The listing builds one solid part. Answer for the finished solid, in the listing's coordinates (mm). A direction names the side the tool comes from. Give positions to 0.01 mm unless a question says otherwise; leave off trailing zeros. Order: outer loops, then holes, each group sorted by start corner. A loop starts at its lowest first (then second) coordinate and runs counter-clockwise, first axis right, second up.
```python
from build123d import *

# Parameters (mm, degrees)
F1_DEPTH       = 35
F3_D           = 5
F3_START       = 1.8205079
F3_CBORE_D     = 10
F3_CBORE_DEPTH = 8
F4_W           = 22.5
F4_H           = 2
F5_DEPTH       = 25
F6_R           = 6
F7_DEPTH       = 8


with BuildPart() as f1:
    # F0 (on Top) → F1 (new body, symmetric)
    with BuildSketch(Plane.XY):
        with BuildLine():
            ThreePointArc((-17.3192642082, 2.5086026559), (17.5, 0), (-17.3192642082, -2.5086026559))
            Line((-17.3192642082, -2.5086026559), (-28.1192642082, -2.5086026559))
            Line((-28.1192642082, -2.5086026559), (-28.1192642082, -10.9086026559))
            ThreePointArc((-28.1192642082, -10.9086026559), (-25.7761184577, -16.5654569054), (-20.1192642082, -18.9086026559))
            Line((-20.1192642082, -18.9086026559), (-7.9192642082, -18.9086026559))
            ThreePointArc((-7.9192642082, -18.9086026559), (20.5, 0), (-7.9192642082, 18.9086026559))
            Line((-7.9192642082, 18.9086026559), (-20.1192642082, 18.9086026559))
            ThreePointArc((-20.1192642082, 18.9086026559), (-25.7761184577, 16.5654569054), (-28.1192642082, 10.9086026559))
            Line((-28.1192642082, 10.9086026559), (-28.1192642082, 2.5086026559))
            Line((-28.1192642082, 2.5086026559), (-17.3192642082, 2.5086026559))
        make_face()
    extrude(amount=F1_DEPTH, both=True)

    # F3 (through all)
    # its depths count from where the whole tool has entered the part; down to there all is cleared
    with Locations(Plane.XZ.offset(18.9086026559).offset(-F3_START)):
        with Locations((-20.2, 24.25), (-20.2, 9.25), (-20.2, -9.25), (-20.2, -24.25)):
            CounterBoreHole(F3_D / 2, F3_CBORE_D / 2, F3_CBORE_DEPTH)

    # F4 (on Front) → F5 (cut, symmetric)
    with BuildSketch(Plane.XZ):
        with Locations((-11.25, 0)):
            Rectangle(F4_W, F4_H)
    extrude(amount=F5_DEPTH, both=True, mode=Mode.SUBTRACT)

    # F6 (on Top) → F7 (cut)
    with BuildSketch(Plane.XY):
        with Locations((0, -25)):
            Circle(F6_R)
        with Locations((17.6776695297, -17.6776695297)):
            Circle(F6_R)
        with Locations((25, 0)):
            Circle(F6_R)
        with Locations((17.6776695297, 17.6776695297)):
            Circle(F6_R)
        with Locations((0, 25)):
            Circle(F6_R)
    extrude(amount=-F7_DEPTH, mode=Mode.SUBTRACT)


solid = f1.part
```
1) Find section C-C (y = 0). Write down the section's boundary in (x, z), then the cut area to 3 significant figures.
Geometry says:
outline: (17.5, -35) - (20.5, -35) - (20.5, -8) - (19, -8) - (19, 0) - (20.5, 0) - (20.5, 35) - (17.5, 35) - close
area: 198 mm2
2) A tool of negligible diameter and unlimited length cuts with its end or side. For faces 1 (the flat face through (20, 0, -8)), 2 (the cylindrical face through (13.4, 13.47, -3.94)), 3 (the cylindrical face through (-15.581, -14.067, 22.335)), from which of +Z, -Z, +X, -X, +Y, -Y can it reach the whole face along a straight path? Write none if from no direction.
Geometry says:
face 1: +X
face 2: +X, +Y
face 3: -Y
3) Find section D-D (z = 9.25). Write down the section's boundary in (x, y), then the cut area to 3 significant figures.
Geometry says:
outline: (-28.12, -10.91) arc R8 ccw to (-25.2, -17.09) - (-25.2, -9.09) - (-22.7, -9.09) - (-22.7, -2.51) - (-28.12, -2.51) - close; (-28.12, 2.51) - (-22.7, 2.51) - (-22.7, 18.48) arc R8 ccw to (-28.12, 10.91) - close; (-17.7, -9.09) - (-15.2, -9.09) - (-15.2, -18.91) - (-7.92, -18.91) arc R20.5 ccw (long way) to (-7.92, 18.91) - (-17.7, 18.91) - (-17.7, 2.51) - (-17.32, 2.51) arc R17.5 cw (long way) to (-17.32, -2.51) - (-17.7, -2.51) - close
area: 487 mm2
4) Find section B-B (x = -11). Write down the section's boundary in (y, z).
Geometry says:
outline: (-18.91, -35) - (-13.61, -35) - (-13.61, -1) - (-18.91, -1) - close; (-18.91, 1) - (-13.61, 1) - (-13.61, 35) - (-18.91, 35) - close; (13.61, -35) - (18.91, -35) - (18.91, -1) - (13.61, -1) - close; (13.61, 1) - (18.91, 1) - (18.91, 35) - (13.61, 35) - close
5) For a pull along Z with two mould halves and no side action, classify faces 4 (the flat face through (-14, 18.909, -18)), 5 (the flat face through (-15, 9.4, -35)), 6 (the flat face through (0, 18.6, 0.2)) as +Z half, -Z half, draft (parallel to the pull), parting line (faces both ways), or undercut.
Geometry says:
face 4: draft
face 5: -Z half
face 6: undercut
6) Straight lines are drawn through the part: probe 1 along Z at (x, y) = (-20.2, 11.25); probe 2 along Z at (x, y) = (-20.2, -13.25); probe 3 along Z at (x, y) = (-17, 8). For each, find the intervals that lie inside material, in ascending order.
Geometry says:
probe 1: z = -35 to -26.75, -21.75 to -11.75, -6.75 to -1, 1 to 6.75, 11.75 to 21.75, 26.75 to 35
probe 2: z = -35 to -29.25, -19.25 to -14.25, -4.25 to -1, 1 to 4.25, 14.25 to 19.25, 29.25 to 35
probe 3: z = -35 to -1, 1 to 35
7) Given P1, Ø3.5, axis at x = -14, z = -12, coming from the -Y side; P2, Ø3, axis at x = -20.2, z = 9.25, coming from the -Y side; P3, Ø1.5, axis at y = -10, z = -6, coming from the +X side; P4, Ø11.5, axis at x = -20.2, z = -9.25, coming from the +Y side, each flat-ended and moving along its own axis, determine where each tip first touches the part or whether it passes through.
Geometry says:
P1: stops at y = -18.91
P2: passes through
P3: stops at x = 18.29
P4: stops at y = 18.91
8) Find section A-A (z = -17). Write down the section's boundary in (x, y), then the cut area to 3 significant figures.
Geometry says:
outline: (-28.12, -10.91) arc R8 ccw to (-20.12, -18.91) - (-7.92, -18.91) arc R20.5 ccw (long way) to (-7.92, 18.91) - (-20.12, 18.91) arc R8 ccw to (-28.12, 10.91) - (-28.12, 2.51) - (-17.32, 2.51) arc R17.5 cw (long way) to (-17.32, -2.51) - (-28.12, -2.51) - close
area: 697 mm2
